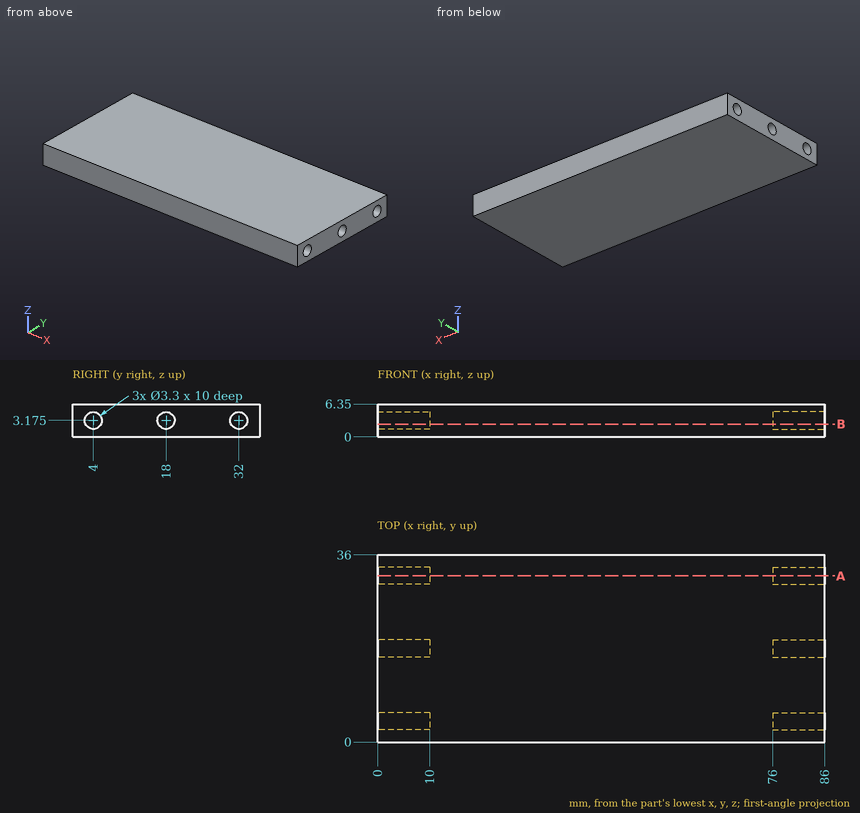
Geometry check sheet. Reference: drawing and pictorial views, mm from the part's lowest x, y, z. Give positions to 0.01 mm unless a question says otherwise; leave off trailing zeros. Order: outer loops, then holes, each group sorted by start corner. A loop starts at its lowest first (then second) coordinate and runs counter-clockwise, first axis right, second up. Notation, with made-up numbers: M 37.5,-33.75 L 62.5,-33.75 A26 ccw 62.5,-18.75 Z; hole C -18,32.25 d6. An arc over 180 degrees is marked long. Answer in a Markdown table with one row per item. Add a question column.
Q1. Sectioned sample at B-B, the plane z = 2.5. Record the boundary of the cut face in (x, y).
Q2. Gauge pin test, flat ends, axial feed: pin 1 Ø1 at (y, z) = (31.5, 2.5) entering from -X; pin 2 Ø1 at (y, z) = (17.5, 3.5) entering from +X. Record the tip position at first contact, or that the pin passes through.
Q3. Thickness scan on L1, parallel to Z at x = 5.5, y = 19. Record the ranges inside material, lowest first.
Q4. Sectioned sample at A-A, the plane y = 32. Record the boundary of the cut face in (x, z) (3 decimals), and give its area (3 significant figures).
Verdict:
| question | item | result |
|---|---|---|
| 1 | outline | M 0,0 L 86,0 L 86,2.49 L 76,2.49 L 76,5.51 L 86,5.51 L 86,16.49 L 76,16.49 L 76,19.51 L 86,19.51 L 86,30.49 L 76,30.49 L 76,33.51 L 86,33.51 L 86,36 L 0,36 L 0,33.51 L 10,33.51 L 10,30.49 L 0,30.49 L 0,19.51 L 10,19.51 L 10,16.49 L 0,16.49 L 0,5.51 L 10,5.51 L 10,2.49 L 0,2.49 Z |
| 2 | pin 1 | x = 10 |
| 2 | pin 2 | x = 76 |
| 3 | L1 | 0 to 1.86, 4.49 to 6.35 |
| 4 | outline | M 0,0 L 86,0 L 86,1.525 L 76,1.525 L 76,4.825 L 86,4.825 L 86,6.35 L 0,6.35 L 0,4.825 L 10,4.825 L 10,1.525 L 0,1.525 Z |
| 4 | area | 480 mm² |
